Check sheet for the modelled part. Datum: model origin and axes. Units: mm. Give positions to 0.01 mm unless a question says otherwise; leave off trailing zeros. Order: outer loops, then holes, each group sorted by start corner. A loop starts at its lowest first (then second) coordinate and runs counter-clockwise, first axis right, second up.
Item 1: Sectioned sample at A-A on y = 1.4. Record the boundary of the cut face in (x, z), and give its area (3 significant figures).
Item 2: Sectioned sample at B-B on x = 78. Record the boundary of the cut face in (y, z), and give its area (3 significant figures).
Item 3: Material ranges on line 1 along Z through (x, y) = (49.5, 1.6); line 2 along Z through (x, y) = (108, 1.55); line 3 along X through (y, z) = (1.25, -266), recorded low to high.
Item 4: Sectioned sample at C-C on z = -258. Record the boundary of the cut face in (x, y).
from build123d import *

# Parameters (mm, degrees)
BOSS_EXTRUDE1_DEPTH = 2.29
CUT_EXTRUDE1_DEPTH  = 3
FILLET1_R           = 10
FILLET2_R           = 3
SKETCH5_W           = 34.038972109
SKETCH5_H           = 16.711464084
CUT_EXTRUDE3_DEPTH  = 10
SKETCH6_W           = 36.357164771
SKETCH6_H           = 12.163218603
CUT_EXTRUDE4_DEPTH  = 10


with BuildPart() as part:
    # Sketch1 → Boss-Extrude1 (new body)
    with BuildSketch(Plane(origin=(0, 0, 0), x_dir=(1, 0, 0), z_dir=(0, 1, 0))):
        with BuildLine():
            Line((1.5, 297.496218463), (1.5, 271.496218463))
            ThreePointArc((1.5, 271.496218463), (70.269464473, 262.249211634), (134.449071126, 235.872622221))
            Line((134.449071126, 235.872622221), (147.449071126, 258.389282719))
            ThreePointArc((147.449071126, 258.389282719), (76.998665918, 287.362933321), (1.5, 297.496218463))
        make_face()
    extrude(amount=BOSS_EXTRUDE1_DEPTH)

    # Sketch3 → Cut-Extrude1 (cut)
    with BuildSketch(Plane(origin=(0, 2.29, 0), x_dir=(1, 0, 0), z_dir=(0, 1, 0))):
        with BuildLine():
            Line((7.5, 271.396751344), (129.203185143, 238.786481168))
            Line((129.203185143, 238.786481168), (136.70589842, 251.781561758))
            ThreePointArc((136.70589842, 251.781561758), (74.15175015, 276.738099028), (7.5, 286.402177897))
            Line((7.5, 286.402177897), (7.5, 271.396751344))
        make_face()
    extrude(amount=-CUT_EXTRUDE1_DEPTH, mode=Mode.SUBTRACT)

    # Fillet1
    fillet1_edges = [part.edges().sort_by_distance(p)[0] for p in [
        (7.5, 1.145, -286.402177897),
        (136.70589842, 1.145, -251.781561758),
    ]]
    fillet(fillet1_edges, radius=FILLET1_R)

    # Fillet2
    fillet2_edges = [part.edges().sort_by_distance(p)[0] for p in [
        (7.5, 1.145, -271.396751344),
        (129.203185143, 1.145, -238.786481168),
    ]]
    fillet(fillet2_edges, radius=FILLET2_R)

    # Sketch5 → Cut-Extrude3 (cut)
    with BuildSketch(Plane.ZY.offset(-1.5)):
        with Locations((-282.724414262, 1.327160447)):
            Rectangle(SKETCH5_W, SKETCH5_H)
    extrude(amount=-CUT_EXTRUDE3_DEPTH, mode=Mode.SUBTRACT)

    # Sketch6 → Cut-Extrude4 (cut)
    with BuildSketch(Plane(origin=(-1.299038106, 0, -0.75), x_dir=(0.5000000000000013, 0, -0.8660254037844379), z_dir=(0.8660254037844378, 0, 0.5000000000000012))):
        with Locations((285.46076815, 1.026498226)):
            Rectangle(SKETCH6_W, SKETCH6_H)
    extrude(amount=-CUT_EXTRUDE4_DEPTH, mode=Mode.SUBTRACT)


solid = part.part
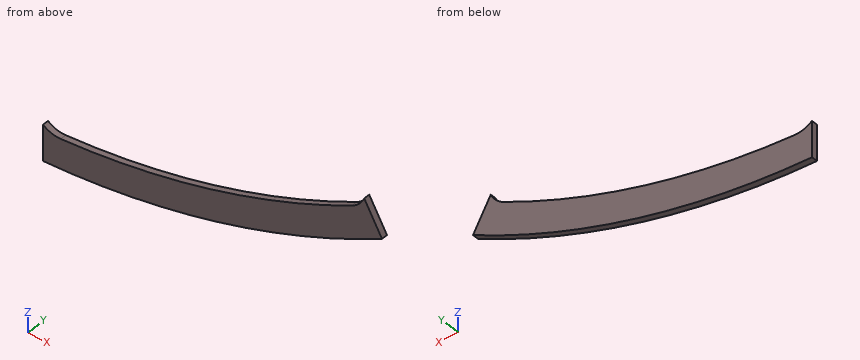
Report:
1. outline: (11.5, -297.28) arc R297.5 ccw to (138.68, -263.2) - (132.01, -251.65) arc R10 cw to (127.26, -256.69) arc R286.5 cw to (18.13, -285.93) arc R10 cw to (11.5, -283.95) - close
1. area: 1,440 mm2
2. outline: (0, -287.09) - (2.29, -287.09) - (2.29, -275.68) - (0, -275.68) - close
2. area: 26.1 mm2
3. line 1: z = -293.35 to -282.19
3. line 2: z = -277.2 to -265.36
3. line 3: x = 106.43 to 133.23
4. outline: (124.57, 0) - (135.68, 0) - (135.68, 2.29) - (124.57, 2.29) - close
